Verification items for the finished model (mm, model axes). Face numbers are marked on the shaded views. A direction names the side the tool comes from. Give positions to 0.01 mm unless a question says otherwise; leave off trailing zeros. Loops run counter-clockwise (first coordinate to the right, second up) from the corner with the lowest first, then second, coordinate; pieces in that order, holes last. Notation, with made-up numbers: (42, -11.5) -> (49, -11.5) arc R28 cw to (49, 27.5) -> close; hole circle Ø10 at (18.25, 60). An arc over 180 degrees is marked (long way). Use one line per item in the form item = value. Start each with the question number.
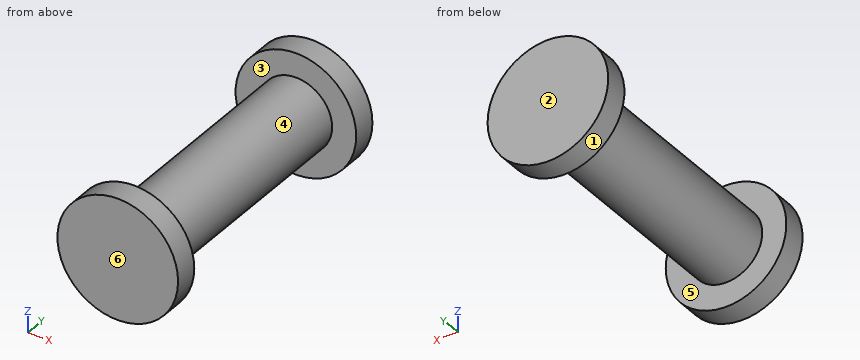
from build123d import *

# Parameters (mm, degrees)
F0_R     = 7.5
F1_DEPTH = 60
F0_R_2   = 12.5
F2_DEPTH = 5
F3_START = 55
F3_DEPTH = 5


with BuildPart() as f1:
    # F0 (on Front) → F1 (new body)
    with BuildSketch(Plane.XZ):
        Circle(F0_R)
    extrude(amount=F1_DEPTH)

    # F0 (on Front) → F2 (join)
    with BuildSketch(Plane.XZ):
        Circle(F0_R_2)
        Circle(F0_R, mode=Mode.SUBTRACT)
    extrude(amount=F2_DEPTH)

    # F0 (on Front) → F3 (join)
    with BuildSketch(Plane.XZ.offset(F3_START)):
        Circle(F0_R_2)
        Circle(F0_R, mode=Mode.SUBTRACT)
    extrude(amount=F3_DEPTH)


solid = f1.part
Item 1: Sectioned sample at C-C, the plane x = -9.75. Enter the section's corners in (y, z), and give its area (3 significant figures).
Item 2: Sectioned sample at A-A, the plane z = 10. Enter the section's corners in (x, y), and give its area (3 significant figures).
Item 3: Draft check along Y on the marked faces 1, 2, 3 and 4. Enter one of: +Y half, -Y half, draft (parallel to the pull), parting line (faces both ways), or undercut.
Item 4: Gauge pin test, flat ends, axial feed: pin 1 Ø2 at (y, z) = (-20.5, -7.5) entering from +X; pin 2 Ø8 at (x, y) = (-3, -46.5) entering from +Z; pin 3 Ø4 at (y, z) = (-38, 2.5) entering from +X. Record the tip position at first contact, or that the pin passes through.
Item 5: Tool access check on the marked faces 5 and 6. Record the directions out of +Z, -Z, +X, -X, +Y, -Y that give a thin tool (end or side, any length) a straight path to the whole face; none if there is none.
Item 6: Sectioned sample at B-B, the plane x = 0. Enter the section's corners in (y, z), and give its area (3 significant figures).
Item 7: Material ranges on line 1 (Y direction, x = -0.75, z = 9.75); line 2 (X direction, y = -4.5, z = 10); line 3 (X direction, y = -19, z = -2.25), recorded low to high.
Item 8: Sectioned sample at D-D, the plane y = -56. Enter the section's corners in (x, z), and give its area (3 significant figures).
Outcome:
q1.outline = (-60, -7.82) -> (-55, -7.82) -> (-55, 7.82) -> (-60, 7.82) -> close; (-5, -7.82) -> (0, -7.82) -> (0, 7.82) -> (-5, 7.82) -> close
q1.area = 156 mm^2
q2.outline = (-7.5, -60) -> (7.5, -60) -> (7.5, -55) -> (-7.5, -55) -> close; (-7.5, -5) -> (7.5, -5) -> (7.5, 0) -> (-7.5, 0) -> close
q2.area = 150 mm^2
q3.face_1 = draft
q3.face_2 = +Y half
q3.face_3 = undercut
q3.face_4 = undercut
q4.pin_1 = 3.74
q4.pin_2 = 7.5
q4.pin_3 = 7.48
q5.face_5 = none
q5.face_6 = +Z, -Z, +X, -X, -Y
q6.outline = (-60, -12.5) -> (-55, -12.5) -> (-55, -7.5) -> (-5, -7.5) -> (-5, -12.5) -> (0, -12.5) -> (0, 12.5) -> (-5, 12.5) -> (-5, 7.5) -> (-55, 7.5) -> (-55, 12.5) -> (-60, 12.5) -> close
q6.area = 1,000 mm^2
q7.line_1 = -60 to -55, -5 to 0
q7.line_2 = -7.5 to 7.5
q7.line_3 = -7.15 to 7.15
q8.outline = circle Ø25 at (0, 0)
q8.area = 491 mm^2
